Read the model definition and answer for the solid it produces. Units are mm, in the model's axes. A direction names the side the tool comes from. Give positions to 0.01 mm unless a question says otherwise; leave off trailing zeros. Write each loop counter-clockwise with the first axis right and the second up, starting at its lowest first coordinate (ties: lowest second). Pieces come first, ordered by that corner, then holes. Notation, with made-up numbers: M 58,-13 L 79,-13 A21 ccw 79,8 Z; hole C 25.25,-1 d10. An arc over 180 degrees is marked long. Answer as CSV lines item,"result". Start each with the question number.
```python
from build123d import *

# Parameters (mm, degrees)
SKETCH1_W           = 27.94
SKETCH1_H           = 6.35
BOSS_EXTRUDE1_DEPTH = 7.9502
SKETCH2_W           = 10.795
SKETCH2_H           = 6.35
BOSS_EXTRUDE2_DEPTH = 151.60625
SKETCH4_R           = 1.5875
CUT_EXTRUDE1_DEPTH  = 161.292682729


with BuildPart() as part:
    # Sketch1 → Boss-Extrude1 (new body)
    with BuildSketch(Plane.XY):
        Rectangle(SKETCH1_W, SKETCH1_H)
    extrude(amount=BOSS_EXTRUDE1_DEPTH)

    # Sketch2 → Boss-Extrude2 (add)
    with BuildSketch(Plane.XY.offset(7.9502)):
        Polygon((-3.302, -3.175), (-3.302, -1.5875), (-6.477, -1.5875), (-6.477, 3.175), (-13.97, 3.175), (-13.97, -3.175), align=None)
        with Locations((8.5725, 0)):
            Rectangle(SKETCH2_W, SKETCH2_H)
    extrude(amount=BOSS_EXTRUDE2_DEPTH)

    # Sketch4 → Cut-Extrude1 (cut, through all)
    with BuildSketch(Plane(origin=(0, 3.175, 0), x_dir=(1, 0, 0), z_dir=(0, 1, 0))):
        with Locations(Location((-8.89, -3.9751, 0), (0, 0, 270))):
            Circle(SKETCH4_R)
        with Locations(Location((8.89, -3.9751, 0), (0, 0, 270))):
            Circle(SKETCH4_R)
    extrude(amount=-CUT_EXTRUDE1_DEPTH, mode=Mode.SUBTRACT)


solid = part.part
```
1. Find section C-C on y = 0.5. Determine the outline of the cut face in (x, z) (1 decimal).
2. For faces 4 (the face through (13.97, 0, 79)), 5 (the face through (3.175, 0, 83)), 6 (the face through (-5, -1.588, 83)), determine the directions among +Z, -Z, +X, -X, +Y, -Y from which every point of the face is accessible in a straight line to the end or side of a thin tool.
3. Find the intervals of material crossed by line 1 (X direction, y = -2.5, z = 113) (3 decimals); line 2 (X direction, y = -0.5, z = 75) (3 decimals); line 3 (Y direction, x = -3.5, z = 107.5) (1 decimal), in increasing order. Write a range as [from, to].
4. Find section A-A on z = 19.5. Determine the outline of the cut face in (x, y) (1 decimal).
5. Find section D-D on x = 0.75. Determine the outline of the cut face in (y, z) (3 decimals).
6. Determine the mould class of faces 1 (the face through (-7.817, 0.044, 2.805)), 2 (the face through (8, 0, 159.556)), 3 (the face through (-13.97, 0, 79)) for opening direction Z: +Z half, -Z half, draft (parallel to the pull), parting line (faces both ways), or undercut.
7. Given pin 1 (1 mm diameter, centred on x = -5.5, z = 98, fed in from +Y); pin 2 (1.9 mm diameter, centred on x = -8.89, z = 3.98, fed in from -Y), each flat-ended and moving along its own axis, determine where each tip first touches the part or whether it passes through.
8. Find section B-B on x = 8.89. Determine the outline of the cut face in (y, z) (3 decimals), then the cut area to 3 significant figures.
Computed:
1,outline,"M -14,0 L 14,0 L 14,159.6 L 3.2,159.6 L 3.2,8 L -6.5,8 L -6.5,159.6 L -14,159.6 Z; hole C -8.9,4 d3.2; hole C 8.9,4 d3.2"
2,face 4,"+Z, -Z, +X, +Y, -Y"
2,face 5,"+Z, +Y, -Y"
2,face 6,"+Z, +Y"
3,line 1,"x = [-13.97, -3.302], [3.175, 13.97]"
3,line 2,"x = [-13.97, -6.477], [3.175, 13.97]"
3,line 3,"y = [-3.2, -1.6]"
4,outline,"M -14,-3.2 L -3.3,-3.2 L -3.3,-1.6 L -6.5,-1.6 L -6.5,3.2 L -14,3.2 Z; M 3.2,-3.2 L 14,-3.2 L 14,3.2 L 3.2,3.2 Z"
5,outline,"M -3.175,0 L 3.175,0 L 3.175,7.95 L -3.175,7.95 Z"
6,face 1,"undercut"
6,face 2,"+Z half"
6,face 3,"draft"
7,pin 1,"stops at y = -1.59"
7,pin 2,"passes through"
8,outline,"M -3.175,0 L 3.175,0 L 3.175,2.388 L -3.175,2.388 Z; M -3.175,5.563 L 3.175,5.563 L 3.175,159.556 L -3.175,159.556 Z"
8,area,"993 mm^2"
